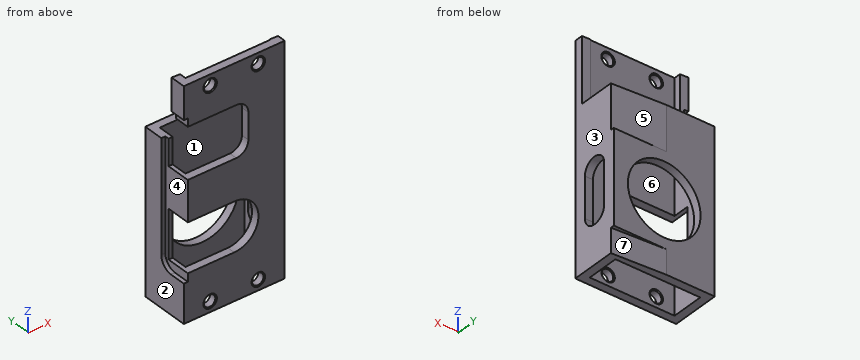
from build123d import *

# Parameters (mm, degrees)
SKETCH_1_W                   = 25
SKETCH_1_H                   = 12
SKETCH_1_W_2                 = 21
SKETCH_1_H_2                 = 8
EXTRUDE_1_DEPTH              = 56
CUT_EXTRUDE_1_REACH          = 14
SKETCH_2_R                   = 9
HOLE_WIZARD_4_401_AT_2_COUNT = 2
HOLE_WIZARD_4_401_AT_2_PITCH = 50.8
HOLE_WIZARD_4_401_AT_3_COUNT = 2
HOLE_WIZARD_4_401_AT_3_PITCH = 52.184323316
HOLE_WIZARD_4_401_AT_4_COUNT = 2
HOLE_WIZARD_4_401_AT_4_PITCH = 11.94
CUT_EXTRUDE_2_DEPTH          = 6
CUT_EXTRUDE_4_DEPTH          = 1
CUT_EXTRUDE_8_REACH          = 27
CUT_EXTRUDE_9_DEPTH          = 6
CUT_EXTRUDE_START            = -56
CUT_EXTRUDE_10_DEPTH         = 27
SKETCH_15_W                  = 30.69445118
SKETCH_15_H                  = 18.97035636
CUT_EXTRUDE_11_DEPTH         = 9


with BuildPart() as part:
    # Sketch 1 → Extrude 1 (new body)
    with BuildSketch(Plane.XY):
        Rectangle(SKETCH_1_W, SKETCH_1_H)
        Rectangle(SKETCH_1_W_2, SKETCH_1_H_2, mode=Mode.SUBTRACT)
    extrude(amount=EXTRUDE_1_DEPTH)

    # Sketch 2 → Cut-Extrude 1 (cut, up to next)
    with BuildSketch(Plane(origin=(0, 6, 0), x_dir=(1, 0, 0), z_dir=(0, 1, 0)), mode=Mode.PRIVATE) as cut_extrude_1_sk1:
        with Locations((0, -17.5)):
            Circle(SKETCH_2_R)
    cut_extrude_1_tool1 = extrude(cut_extrude_1_sk1.sketch, amount=-CUT_EXTRUDE_1_REACH, mode=Mode.PRIVATE) & part.part
    add(cut_extrude_1_tool1.solids().sort_by_distance((0, 6, 17.5))[0], mode=Mode.SUBTRACT)

    # Sketch 3 → Hole Wizard 4-401 (revolve, cut)
    with BuildSketch(Plane(origin=(5.97, -6, 53.37), x_dir=(0, 0, -1), z_dir=(1, 0, 0))):
        Polygon((0, 0), (0, 2), (1.6764, 2), (1.4224, 1.822147285), (1.4224, 0.177852715), (1.6764, 0), align=None)
    hole_wizard_4_401 = revolve(axis=Axis((5.97, -12.35, 53.37), (0, 1, 0)), mode=Mode.SUBTRACT)

    # Hole Wizard 4-401 at 2: Hole Wizard 4-401 ×2
    with Locations(*[(0, 0, -i * HOLE_WIZARD_4_401_AT_2_PITCH) for i in range(1, HOLE_WIZARD_4_401_AT_2_COUNT)]):
        add(hole_wizard_4_401, mode=Mode.SUBTRACT)

    # Hole Wizard 4-401 at 3: Hole Wizard 4-401 ×2
    with Locations(*[Vector(-0.228804347, 0, -0.973472429) * (i * HOLE_WIZARD_4_401_AT_3_PITCH) for i in range(1, HOLE_WIZARD_4_401_AT_3_COUNT)]):
        add(hole_wizard_4_401, mode=Mode.SUBTRACT)

    # Hole Wizard 4-401 at 4: Hole Wizard 4-401 ×2
    with Locations(*[(-i * HOLE_WIZARD_4_401_AT_4_PITCH, 0, 0) for i in range(1, HOLE_WIZARD_4_401_AT_4_COUNT)]):
        add(hole_wizard_4_401, mode=Mode.SUBTRACT)

    # Sketch 5 → Cut-Extrude 2 (cut)
    with BuildSketch(Plane.XZ.offset(6)):
        with BuildLine():
            Line((-12.5, 11.5), (0, 11.5))
            ThreePointArc((0, 11.5), (6, 17.5), (0, 23.5))
            Line((0, 23.5), (-12.5, 23.5))
            Line((-12.5, 23.5), (-12.5, 11.5))
        make_face()
        with BuildLine():
            Line((-12.5, 46), (0.5, 46))
            ThreePointArc((0.5, 46), (2.621320344, 45.121320344), (3.5, 43))
            Line((3.5, 43), (3.5, 36.5))
            ThreePointArc((3.5, 36.5), (2.621320344, 34.378679656), (0.5, 33.5))
            Line((0.5, 33.5), (-12.5, 33.5))
            Line((-12.5, 33.5), (-12.5, 46))
        make_face()
    extrude(amount=-CUT_EXTRUDE_2_DEPTH, mode=Mode.SUBTRACT)

    # Sketch 8 → Cut-Extrude 4 (cut)
    with BuildSketch(Plane.ZY.offset(12.5)):
        with BuildLine():
            Line((9.5, -6), (9.5, -2))
            ThreePointArc((9.5, -2), (10.378679656, 0.121320344), (12.5, 1))
            Line((12.5, 1), (45, 1))
            ThreePointArc((45, 1), (47.121320344, 0.121320344), (48, -2))
            Line((48, -2), (48, -6))
            Line((48, -6), (9.5, -6))
        make_face()
    extrude(amount=-CUT_EXTRUDE_4_DEPTH, mode=Mode.SUBTRACT)

    # Sketch 13 → Cut-Extrude 8 (cut, up to next)
    with BuildSketch(Plane(origin=(12.5, 0, 0), x_dir=(0, 0, -1), z_dir=(1, 0, 0)), mode=Mode.PRIVATE) as cut_extrude_8_sk1:
        with BuildLine():
            Line((-22.5, 3), (-12.5, 3))
            ThreePointArc((-12.5, 3), (-9.5, 0), (-12.5, -3))
            Line((-12.5, -3), (-22.5, -3))
            ThreePointArc((-22.5, -3), (-25.5, 0), (-22.5, 3))
        make_face()
    cut_extrude_8_tool1 = extrude(cut_extrude_8_sk1.sketch, amount=-CUT_EXTRUDE_8_REACH, mode=Mode.PRIVATE) & part.part
    add(cut_extrude_8_tool1.solids().sort_by_distance((12.5, 0, 17.5))[0], mode=Mode.SUBTRACT)

    # Sketch 14 → Cut-Extrude 9 (cut)
    with BuildSketch(Plane(origin=(0, 0, 0), x_dir=(-1, 0, 0), z_dir=(0, 0, -1))):
        Polygon((-12.5, 6), (-12.5, 5.083085997), (0.612481145, 6), align=None)
    extrude(amount=-CUT_EXTRUDE_9_DEPTH, mode=Mode.SUBTRACT)

    # Sketch 14_3 → Cut-Extrude 10 (cut)
    with BuildSketch(Plane(origin=(0, 0, 0), x_dir=(-1, 0, 0), z_dir=(0, 0, -1)).offset(CUT_EXTRUDE_START)):
        Polygon((-12.5, 6), (-12.5, 5.083085997), (0.612481145, 6), align=None)
    extrude(amount=CUT_EXTRUDE_10_DEPTH, mode=Mode.SUBTRACT)

    # Sketch 15 → Cut-Extrude 11 (cut)
    with BuildSketch(Plane(origin=(0.414538991, 5.928183756, 0), x_dir=(0.99756405, -0.069756474, 0), z_dir=(0.069756474, 0.99756405, 0))):
        with Locations((-0.241417032, -49.48517818)):
            Rectangle(SKETCH_15_W, SKETCH_15_H)
    extrude(amount=-CUT_EXTRUDE_11_DEPTH, mode=Mode.SUBTRACT)


solid = part.part
Build history of the part. All positions in model axes, mm. Face numbers are marked on the shaded views. A direction names the side the tool comes from. Give positions to 0.01 mm unless a question says otherwise; leave off trailing zeros. Write each loop counter-clockwise with the first axis right and the second up, starting at its lowest first coordinate (ties: lowest second). Pieces come first, ordered by that corner, then holes. Notation, with made-up numbers: (-27.75, 14) - (29.25, 14) arc R15 ccw to (29.25, 31) - close; hole circle Ø1 at (-13, 47.5). An arc over 180 degrees is marked (long way). Use one line per item in the form item = value. Start each with the question number.
1. Drop flat-ended pins along their axis: pin 1 Ø2 at (y, z) = (-5, 41) entering from -X; pin 2 Ø0.5 at (y, z) = (-3.5, 51) entering from +X; pin 3 Ø1.1 at (x, z) = (-12, 22) entering from -Y. Give the stop position or say it passes through.
2. Band-saw the part on D-D on x = 11.25. Write the cut outline in (y, z), plus the area to 3 significant figures.
3. Two-plate mould, pull along X, no slides. Class the marked faces 1, 2 and 3: released by +X, released by -X, zero draft, split by the parting line, or undercut.
4. Band-saw the part on A-A on z = 53.37. Write the cut outline in (x, y).
5. 3-axis set-ups, long thin cutter, end or side, ignore diameter. For the marked faces 4, 5, 6 and 7: which of +Z, -Z, +X, -X, +Y, -Y reach the whole face in a straight line?
6. Band-saw the part on C-C on y = -0.5. Write the cut outline in (x, z).
7. Probe line 1 (X direction, y = -5.15, z = 2.57); line 2 (Z direction, x = -5.97, y = -5.4); line 3 (Z direction, x = 0, y = 5.15). List the from-to ranges inside material, lowest first. Write a range as [from, to].
8. Band-saw the part on B-B on z = 2.57. Write the cut outline in (x, y), plus the area to 3 significant figures.
Conclusion:
q1.pin_1 = 3.5
q1.pin_2 = -10.5
q1.pin_3 = 0
q2.outline = (-6, 0) - (5.17, 0) - (5.17, 6) - (6, 6) - (6, 29) - (5.17, 29) - (5.17, 40) - (-3.85, 40) - (-3.85, 56) - (-6, 56) - close; hole (-3, 12.5) arc R3 ccw to (3, 12.5) - (3, 22.5) arc R3 ccw to (-3, 22.5) - close
q2.area = 412 mm²
q3.face_1 = undercut
q3.face_2 = released by -X
q3.face_3 = released by +X
q4.outline = (-12.5, -6) - (-7.65, -6) - (-7.39, -5.82) - (-7.39, -4.18) - (-7.65, -4) - (-10.5, -4) - (-10.5, -2.33) - (-12.5, -2.19) - close; (-4.55, -5.82) - (-4.29, -6) - (4.29, -6) - (4.55, -5.82) - (4.55, -4.18) - (4.29, -4) - (-4.29, -4) - (-4.55, -4.18) - close; (7.39, -5.82) - (7.65, -6) - (12.5, -6) - (12.5, -3.94) - (10.5, -3.8) - (10.5, -4) - (7.65, -4) - (7.39, -4.18) - close
q5.face_4 = -X, -Y
q5.face_5 = +Z, +X, +Y
q5.face_6 = +Z, -Z
q5.face_7 = -Z, +X, +Y
q6.outline = (-12.5, 0) - (-10.5, 0) - (-10.5, 11.5) - (-11.5, 11.5) - (-11.5, 9.9) - (-12.5, 9.9) - close; (-11.5, 23.5) - (-10.5, 23.5) - (-10.5, 33.5) - (-11.5, 33.5) - close; (10.5, 0) - (12.5, 0) - (12.5, 9.54) - (10.5, 9.54) - close; (10.5, 25.46) - (12.5, 25.46) - (12.5, 40) - (10.5, 40) - close
q7.line_1 = [-12.5, -7.39], [-4.55, 4.55], [7.39, 12.5]
q7.line_2 = [0, 1.15], [3.99, 11.5], [23.5, 33.5], [46, 51.95], [54.79, 56]
q7.line_3 = [0, 8.5], [26.5, 40]
q8.outline = (-12.5, -6) - (-7.65, -6) - (-7.39, -5.82) - (-7.39, -4.18) - (-7.65, -4) - (-10.5, -4) - (-10.5, 4) - (10.5, 4) - (10.5, -4) - (7.65, -4) - (7.39, -4.18) - (7.39, -5.82) - (7.65, -6) - (12.5, -6) - (12.5, 5.08) - (-0.61, 6) - (-12.5, 6) - close; (-4.55, -5.82) - (-4.29, -6) - (4.29, -6) - (4.55, -5.82) - (4.55, -4.18) - (4.29, -4) - (-4.29, -4) - (-4.55, -4.18) - close
q8.area = 114 mm²
